Check sheet for the modelled part. Datum: model origin and axes. Units: mm. Face numbers are marked on the shaded views. A direction names the side the tool comes from. Round coordinates to 2 decimals unless told otherwise and drop trailing zeros. Order: outer loops, then holes, each group sorted by start corner. A loop starts at its lowest first (then second) coordinate and runs counter-clockwise, first axis right, second up. Notation, with made-up numbers: (86, 2) -> (90, 2) arc R22 cw to (90, 24) -> close; hole circle Ø11 at (9, 27.5). An arc over 180 degrees is marked (long way). Use CSV: the item, a comma, the result in double quotes.
```python
from build123d import *

# Parameters (mm, degrees)
F0_R     = 88.9
F0_R_2   = 1.5875
F1_DEPTH = 6.35
F2_DEPTH = 25.4


with BuildPart() as f1:
    # F0 (on Front) → F1 (new body)
    with BuildSketch(Plane.XZ):
        with BuildLine():
            ThreePointArc((-21.163168, 66.848182), (-20.535293, 70.811884), (-24.291636, 72.224348))
            ThreePointArc((-24.291636, 72.224348), (-66.115053, 37.884558), (-74.594011, -15.561926))
            ThreePointArc((-74.594011, -15.561926), (-71.46933, -18.088469), (-68.371234, -15.529397))
            ThreePointArc((-68.371234, -15.529397), (-47.541779, 8.338621), (-16.441051, 2.314237))
            ThreePointArc((-16.441051, 2.314237), (-14.081698, 1.024394), (-11.400071, 0.826612))
            ThreePointArc((-11.400071, 0.826612), (-6.789469, 3.932244), (-6.390105, 9.476891))
            ThreePointArc((-6.390105, 9.476891), (-7.914512, 11.721964), (-10.237, 13.12561))
            ThreePointArc((-10.237, 13.12561), (-31.113041, 36.852188), (-21.163168, 66.848182))
        make_face()
        Circle(F0_R)
        with Locations((-59.033186, -57.70256)):
            Circle(F0_R_2, mode=Mode.SUBTRACT)
        with Locations((-38.312825, -73.120653)):
            Circle(F0_R_2, mode=Mode.SUBTRACT)
        with Locations((-13.842137, -81.381188)):
            Circle(F0_R_2, mode=Mode.SUBTRACT)
        with Locations((-73.974968, -36.636138)):
            Circle(F0_R_2, mode=Mode.SUBTRACT)
        with Locations((-81.675565, -11.983515)):
            Circle(F0_R_2, mode=Mode.SUBTRACT)
        with Locations((11.983515, -81.675565)):
            Circle(F0_R_2, mode=Mode.SUBTRACT)
        with Locations((36.636138, -73.974968)):
            Circle(F0_R_2, mode=Mode.SUBTRACT)
        with Locations((57.70256, -59.033186)):
            Circle(F0_R_2, mode=Mode.SUBTRACT)
        with Locations((73.120653, -38.312825)):
            Circle(F0_R_2, mode=Mode.SUBTRACT)
        with Locations((81.381188, -13.842137)):
            Circle(F0_R_2, mode=Mode.SUBTRACT)
        with Locations((-81.381188, 13.842137)):
            Circle(F0_R_2, mode=Mode.SUBTRACT)
        with Locations((-73.120653, 38.312825)):
            Circle(F0_R_2, mode=Mode.SUBTRACT)
        with Locations((-57.70256, 59.033186)):
            Circle(F0_R_2, mode=Mode.SUBTRACT)
        with Locations((-36.636138, 73.974968)):
            Circle(F0_R_2, mode=Mode.SUBTRACT)
        with Locations((-11.983515, 81.675565)):
            Circle(F0_R_2, mode=Mode.SUBTRACT)
        with BuildLine():
            ThreePointArc((-24.291636, 72.224348), (44.471437, 61.876743), (76.2, 0))
            ThreePointArc((76.2, 0), (7.822288, -75.797439), (-74.594011, -15.561926))
            ThreePointArc((-74.594011, -15.561926), (-66.115053, 37.884558), (-24.291636, 72.224348))
        make_face(mode=Mode.SUBTRACT)
        with Locations((81.675565, 11.983515)):
            Circle(F0_R_2, mode=Mode.SUBTRACT)
        with Locations((73.974968, 36.636138)):
            Circle(F0_R_2, mode=Mode.SUBTRACT)
        with Locations((13.842137, 81.381188)):
            Circle(F0_R_2, mode=Mode.SUBTRACT)
        with Locations((38.312825, 73.120653)):
            Circle(F0_R_2, mode=Mode.SUBTRACT)
        with Locations((59.033186, 57.70256)):
            Circle(F0_R_2, mode=Mode.SUBTRACT)
    extrude(amount=F1_DEPTH)

    # F0 (on Front) → F2 (join)
    with BuildSketch(Plane.XZ):
        with BuildLine():
            ThreePointArc((-21.163168, 66.848182), (-20.535293, 70.811884), (-24.291636, 72.224348))
            ThreePointArc((-24.291636, 72.224348), (-66.115053, 37.884558), (-74.594011, -15.561926))
            ThreePointArc((-74.594011, -15.561926), (-71.46933, -18.088469), (-68.371234, -15.529397))
            ThreePointArc((-68.371234, -15.529397), (-47.541779, 8.338621), (-16.441051, 2.314237))
            ThreePointArc((-16.441051, 2.314237), (-14.081698, 1.024394), (-11.400071, 0.826612))
            ThreePointArc((-11.400071, 0.826612), (-6.789469, 3.932244), (-6.390105, 9.476891))
            ThreePointArc((-6.390105, 9.476891), (-7.914512, 11.721964), (-10.237, 13.12561))
            ThreePointArc((-10.237, 13.12561), (-31.113041, 36.852188), (-21.163168, 66.848182))
        make_face()
    extrude(amount=F2_DEPTH)


solid = f1.part
```
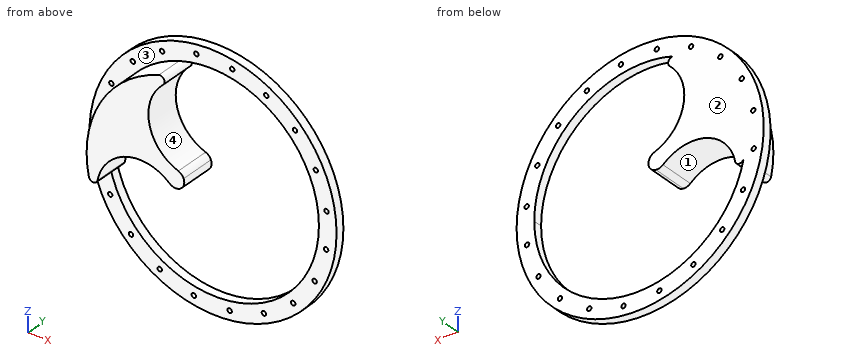
Q1. Access from +Z, -Z, +X, -X, +Y, -Y to the whole of each face (thin tool, end or side, straight path). Record for the marked faces 1 and 2.
Result sheet:
face 1,"+Y, -Y"
face 2,"+Z, -Z, +X, -X, +Y"
Q2. Mould release check, pull along X, two halves, no side actions. Record for the marked faces 3 and 4: pulls with the +X half, pulls with the -X half, needs draft (parallel to the pull), parting line crosses it, or undercut.
Result sheet:
face 3,"needs draft"
face 4,"undercut"
Q3. Scan lines: L1, parallel to X at y = -3.5, z = 34; L2, parallel to Y at x = -50.5, z = 73; L3, parallel to Z at x = -27, y = -9.5. Record each from-to range of solid material in increasing order.
Result sheet:
L1,"x = -82.14 to -30.39, 68.19 to 82.14"
L2,"y = -6.35 to 0"
L3,"z = 8.37 to 26.47, 59.89 to 71.26"
Q4. Sectioned sample at A-A, the plane x = 0. Enter the section's corners in (y, z), then the cut area to 3 significant figures.
Result sheet:
outline,"(-6.35, -88.9) -> (0, -88.9) -> (0, -76.2) -> (-6.35, -76.2) -> close; (-6.35, 76.2) -> (0, 76.2) -> (0, 88.9) -> (-6.35, 88.9) -> close"
area,"161 mm^2"
Q5. Sectioned sample at D-D, the plane z = 6. Enter the section's corners in (x, y).
Result sheet:
outline,"(-88.7, -6.35) -> (-75.96, -6.35) -> (-75.96, -25.4) -> (-52.76, -25.4) -> (-52.76, 0) -> (-88.7, 0) -> close; (-21.69, -25.4) -> (-6.03, -25.4) -> (-6.03, 0) -> (-21.69, 0) -> close; (75.96, -6.35) -> (88.7, -6.35) -> (88.7, 0) -> (75.96, 0) -> close"
Q6. Go/stop test with flat-tipped pins: pin 1 (12 mm diameter, centred on y = -19.5, z = 59.5, fed in from +X); pin 2 (4 mm diameter, centred on x = -59.03, z = -57.7, fed in from -Y); pin 3 (2 mm diameter, centred on y = -12, z = 17, fed in from +X). Record where each tip stops, or that it passes through.
Result sheet:
pin 1,"stops at x = -22.58"
pin 2,"stops at y = -6.35"
pin 3,"stops at x = -16.41"
Q7. Sectioned sample at B-B, the plane z = -32.5. Enter the section's corners in (x, y), then the cut area to 3 significant figures.
Result sheet:
outline,"(-82.75, -6.35) -> (-68.92, -6.35) -> (-68.92, 0) -> (-82.75, 0) -> close; (68.92, -6.35) -> (82.75, -6.35) -> (82.75, 0) -> (68.92, 0) -> close"
area,"176 mm^2"
Q8. Sectioned sample at C-C, the plane y = -11.25. Enter the section's corners in (x, z) (3 decimals).
Result sheet:
outline,"(-74.594, -15.562) arc R3.175 ccw to (-68.371, -15.529) arc R31.75 cw to (-16.441, 2.314) arc R6.35 ccw to (-11.4, 0.827) arc R6.35 ccw to (-6.39, 9.477) arc R6.35 ccw to (-10.237, 13.126) arc R31.75 cw to (-21.163, 66.848) arc R3.175 ccw to (-24.292, 72.224) arc R76.2 ccw to start"
